Model file for the job. Use its own axes, mm. A direction names the side the tool comes from. Coordinates: 2 decimals unless noted, no trailing zeros. Order: outer loops, then holes, each group sorted by start corner. A loop starts at its lowest first (then second) coordinate and runs counter-clockwise, first axis right, second up. Notation, with made-up numbers: M 49.5,87.5 L 61.5,87.5 A14 cw 61.5,99.5 Z; hole C 16,-9 d6. An arc over 180 degrees is marked long. Return JSON: item names as keys, results as strings.
Autodesk Inventor part; units mm, degrees
ref_plane "YZ Plane" through (0, 0, 0) normal (1, 0, 0) x (0, 1, 0)
ref_plane "XZ Plane" through (0, 0, 0) normal (0, 1, 0) x (-1, 0, 0)
ref_plane "XY Plane" through (0, 0, 0) normal (0, 0, 1) x (1, 0, 0)
sketch "Sketch1" plane through (0, 0, 0) normal (0, 1, 0) x (-1, 0, 0)
  line L0 (0, 0) -> (-37, 0)
  line L1 (-37, 0) -> (-37, 37)
  line L2 (-37, 37) -> (0, 37)
  line L3 (0, 37) -> (0, 0)
  circle A0 centre (-18.5, 18.5) radius 15.5
  point P0 (-18.5, 0)
  dimension "d0" = 37
  dimension "d1" = 37
  dimension "d2" = 18.5
  dimension "d3" = 18.5
  dimension "d4" = 31
extrude "Extrusion1" add sketch "Sketch1" against normal blind 35
sketch "Sketch3" plane through (0, 0, 37) normal (0, 0, 1) x (1, 0, 0)
  circle A0 centre (18.5, -10) radius 4.5
  line L0 (37, 0) -> (37, -35)
  point P0 (0, 0)
  dimension "d8" = 9
  dimension "d18" = 18.5
extrude "Extrusion2" cut sketch "Sketch3" along normal mid plane 5
sketch "Sketch4" plane through (37, 0, 0) normal (0, 0, -1) x (-1, 0, 0)
  circle A0 centre (18.5, -10) radius 4.5
  circle A1 centre (18.5, -10) radius 2.5
  point P0 (37, 0)
  dimension "d11" = 5
extrude "Extrusion3" cut sketch "Sketch4" against normal blind 5 contours A1
sketch "Sketch5" plane through (0, 0, 37) normal (0, 0, 1) x (1, 0, 0)
  line L0 (37, 0) -> (0, 0)
  line L1 (0, -35) -> (37, -35)
  line L2 (0, 0) -> (37, 0)
  line L3 (37, 0) -> (37, -35)
  line L4 (37, -35) -> (0, -35)
  line L5 (0, -35) -> (0, 0)
  line L6 (0, 0) -> (0, -35)
  line L7 (0, 0) -> (37, 0)
  line L8 (37, 0) -> (37, -35)
  line L9 (37, -35) -> (0, -35)
  line L10 (0, -35) -> (0, 0)
  circle A0 centre (18.5, -25) radius 4.5
  dimension "d19" = 18.5
  dimension "d22" = 10
extrude "Extrusion4" add sketch "Sketch5" along normal blind 2
sketch "Sketch6" plane through (0, 0, 39) normal (0, 0, 1) x (1, 0, 0)
  line L0 (0, 0) -> (0, -35)
  line L1 (0, -35) -> (37, -35)
  line L2 (0, 0) -> (37, 0)
  line L3 (37, 0) -> (37, -35)
  line L4 (37, -35) -> (0, -35)
  line L5 (0, -35) -> (0, 0)
extrude "Extrusion5" add sketch "Sketch6" along normal blind 5
sketch "Sketch7" plane through (0, 0, 44) normal (0, 0, 1) x (1, 0, 0)
  circle A0 centre (18.5, -10) radius 2.5
  line L0 (37, 0) -> (0, 0)
  line L1 (37, -35) -> (37, 0)
  point P0 (18.5, 0)
  dimension "d24" = 5
  dimension "d25" = 10
  dimension "d26" = 18.5
extrude "Extrusion6" cut sketch "Sketch7" against normal through all
sketch "Sketch8" plane through (18.5, -10, 34.5) normal (0, 0, 1) x (1, 0, 0)
  circle A0 centre (0, 0) radius 2.5
  circle A1 centre (0, 0) radius 4.5
  point P0 (-18.5, 10)
extrude "Extrusion7" cut sketch "Sketch8" along normal mid plane 8
equation "\"d0\" = d1"
properties part number "pump mount v04"
Item 1: Saw through at B-B (z = 18.5). Write the cut outline in (x, y), and give its area (3 significant figures).
Check result:
{"outline": "M 0,-35 L 3,-35 L 3,0 L 0,0 Z; M 34,-35 L 37,-35 L 37,0 L 34,0 Z", "area": "210 mm2"}
Item 2: 3-axis set-ups, long thin cutter, end or side, ignore diameter. For faces 1 (the cylindrical face through (15.18, -28.04, 37.99)), 2 (the flat face through (18, -35, 36)): which of +Z, -Z, +X, -X, +Y, -Y reach the whole face in a straight line?
Check result:
{"face 1": "none", "face 2": "+Z, -Z, +X, -X, -Y"}
Item 3: Saw through at D-D (x = 24). Write the cut outline in (y, z).
Check result:
{"outline": "M -35,0 L 0,0 L 0,4.01 L -35,4.01 Z; M -35,32.99 L 0,32.99 L 0,44 L -35,44 Z"}
Item 4: Wall check: line 1 (Y direction, x = 18.5, z = 38.05); line 2 (Z direction, x = 18.5, y = -26.5); line 3 (X direction, y = -10, z = 35.65). Give the ranges that are in metal, low to high.
Check result:
{"line 1": "y = -35 to -29.5, -20.5 to -14.5, -5.5 to 0", "line 2": "z = 0 to 3, 34 to 37, 39 to 44", "line 3": "x = 0 to 14, 23 to 37"}
Item 5: Saw through at C-C (y = -10). Write the cut outline in (x, z).
Check result:
{"outline": "M 0,0 L 16,0 L 16,3.2 A15.5 cw 14,33.33 L 14,38.5 L 16,38.5 L 16,44 L 0,44 Z; M 21,0 L 37,0 L 37,44 L 21,44 L 21,38.5 L 23,38.5 L 23,33.33 A15.5 cw 21,3.2 Z"}
Item 6: Saw through at A-A (x = 18.5). Write the cut outline in (y, z).
Check result:
{"outline": "M -35,0 L -12.5,0 L -12.5,3 L -35,3 Z; M -35,34 L -14.5,34 L -14.5,38.5 L -12.5,38.5 L -12.5,44 L -35,44 Z; M -7.5,0 L 0,0 L 0,3 L -7.5,3 Z; M -7.5,38.5 L -5.5,38.5 L -5.5,34 L 0,34 L 0,44 L -7.5,44 Z; hole M -29.5,37 L -20.5,37 L -20.5,39 L -29.5,39 Z"}
Item 7: Pull direction X, two halves, no side cores. Call faces 3 (the flat face through (0, -17, 22)), 4 (the flat face through (18, -17, 44)), 5 (the cylindrical face through (17, -12, 41)): +X half, -X half, draft (parallel to the pull), parting line (faces both ways), or undercut.
Check result:
{"face 3": "-X half", "face 4": "draft", "face 5": "undercut"}
